from build123d import *

# Parameters (mm, degrees)
SKETCH_1_W          = 46
SKETCH_1_H          = 25
EXTRUDE_1_DEPTH     = 1
SKETCH_2_W          = 48
SKETCH_2_H          = 27
EXTRUDE_2_DEPTH     = 1
FILLET_1_R          = 1
SKETCH_3_W          = 34
SKETCH_3_H          = 12
CUT_EXTRUDE_2_DEPTH = 2


with BuildPart() as part:
    # ｽｹｯﾁ1 → ﾎﾞｽ - 押し出し1 (new body)
    with BuildSketch(Plane(origin=(0, 0, 0), x_dir=(1, 0, 0), z_dir=(0, 1, 0))):
        with Locations((-2.865663922, 0.615345108)):
            Rectangle(SKETCH_1_W, SKETCH_1_H)
    extrude(amount=EXTRUDE_1_DEPTH)

    # ｽｹｯﾁ2 → ﾎﾞｽ - 押し出し2 (add)
    with BuildSketch(Plane(origin=(0, 1, 0), x_dir=(1, 0, 0), z_dir=(0, 1, 0))):
        with Locations((-2.865663922, 0.615345108)):
            Rectangle(SKETCH_2_W, SKETCH_2_H)
    extrude(amount=EXTRUDE_2_DEPTH)

    # ﾌｨﾚｯﾄ1
    fillet_1_edges = [part.edges().sort_by_distance(p)[0] for p in [
        (-26.865663922, 1.5, -14.115345108),
        (-26.865663922, 1.5, 12.884654892),
        (21.134336078, 1.5, 12.884654892),
        (21.134336078, 1.5, -14.115345108),
        (-26.865663922, 2, -0.615345108),
        (-2.865663922, 2, 12.884654892),
        (21.134336078, 2, -0.615345108),
        (-2.865663922, 2, -14.115345108),
    ]]
    fillet(fillet_1_edges, radius=FILLET_1_R - 0.0001)  # a hair under: the kernel refuses the full size

    # ｽｹｯﾁ3 → ｶｯﾄ - 押し出し2 (cut)
    with BuildSketch(Plane(origin=(0, 2, 0), x_dir=(1, 0, 0), z_dir=(0, 1, 0))):
        with Locations((0.134336078, -3.584654892)):
            Rectangle(SKETCH_3_W, SKETCH_3_H)
    extrude(amount=-CUT_EXTRUDE_2_DEPTH, mode=Mode.SUBTRACT)


solid = part.part
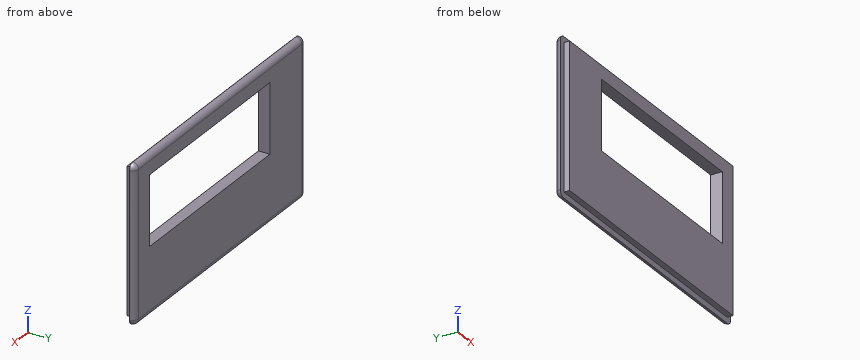
Read the model definition and answer for the solid it produces. Units are mm, in the model's axes. Round coordinates to 2 decimals unless told otherwise and drop trailing zeros. Loops run counter-clockwise (first coordinate to the right, second up) from the corner with the lowest first, then second, coordinate; pieces in that order, holes last.
Q1. Section B-B on y = 0.4 is taken. Write down the section's boundary in (x, z), and give its area (3 significant figures).
Q2. Each of these flat-tipped pins is pushed along its axis until it touches: pin 1 (0.5 mm diameter, centred on x = -1.5, y = 0.5, fed in from -Z); pin 2 (0.8 mm diameter, centred on y = 0.5, z = -3, fed in from -X); pin 3 (0.8 mm diameter, centred on y = 0.5, z = -1.5, fed in from +X). Where does it stop, or does it pass through?
Q3. Consider probe 1 along Z at (x, y) = (13.5, 1.15); probe 2 along X at (y, z) = (1.1, 0.5); probe 3 along Z at (x, y) = (3, 0.9). Determine where each line is inside the solid, lowest interval first.
Output:
1. outline: (-25.87, -13.12) - (20.13, -13.12) - (20.13, 11.88) - (-25.87, 11.88) - close; hole (-16.87, -2.42) - (17.13, -2.42) - (17.13, 9.58) - (-16.87, 9.58) - close
1. area: 742 mm2
2. pin 1: stops at z = -13.12
2. pin 2: stops at x = -25.87
2. pin 3: stops at x = 20.13
3. probe 1: z = -14.1 to -2.42, 9.58 to 12.87
3. probe 2: x = -26.86 to -16.87, 17.13 to 21.13
3. probe 3: z = -13.12 to -2.42, 9.58 to 11.88
